Autodesk Inventor part; units mm, degrees
ref_plane "YZ Plane" through (0, 0, 0) normal (1, 0, 0) x (0, 1, 0)
ref_plane "XZ Plane" through (0, 0, 0) normal (0, 1, 0) x (-1, 0, 0)
ref_plane "XY Plane" through (0, 0, 0) normal (0, 0, 1) x (1, 0, 0)
sketch "Sketch1" plane through (0, 0, 0) normal (0, 1, 0) x (-1, 0, 0)
  line L0 (19.2289, 19.6338) -> (19.2289, -32.3662)
  line L1 (17.2289, -34.3662) -> (-13.7711, -34.3662)
  line L2 (-15.7711, -32.3662) -> (-15.7711, -10.826)
  line L3 (-19.7711, -6.826) -> (-35.887, -6.826)
  line L4 (-37.887, -4.826) -> (-37.887, 10.574)
  line L5 (17.2289, 21.6338) -> (-13.3861, 21.6338)
  line L6 (-14.943, 20.8893) -> (-16.2097, 19.3185)
  line L7 (-17.7665, 18.574) -> (-35.887, 18.574)
  line L8 (-16.8101, 12.574) -> (-36.4101, 12.574)
  line L9 (-36.4101, 12.574) -> (-36.4101, 10.174)
  line L10 (-36.4101, 10.174) -> (-16.8101, 10.174)
  line L11 (-16.8101, 10.174) -> (-16.8101, 12.574)
  arc A0 (19.2289, 19.6338) -> (17.2289, 21.6338) centre (17.2289, 19.6338) ccw
  arc A1 (17.2289, -34.3662) -> (19.2289, -32.3662) centre (17.2289, -32.3662) ccw
  arc A2 (-15.7711, -32.3662) -> (-13.7711, -34.3662) centre (-13.7711, -32.3662) ccw
  arc A3 (-15.7711, -10.826) -> (-19.7711, -6.826) centre (-19.7711, -10.826) ccw
  arc A4 (-37.887, -4.826) -> (-35.887, -6.826) centre (-35.887, -4.826) ccw
  arc A5 (-17.7665, 18.574) -> (-16.2097, 19.3185) centre (-17.7665, 20.574) ccw
  arc A6 (-13.3861, 21.6338) -> (-14.943, 20.8893) centre (-13.3861, 19.6338) ccw
  line L12 (-33.327, 18.574) -> (-41.327, 18.574)
  line L13 (-43.327, 16.574) -> (-43.327, 14.574)
  line L14 (-41.327, 12.574) -> (-39.887, 12.574)
  circle A7 centre (-40.327, 15.574) radius 1.5
  arc A8 (-37.887, 10.574) -> (-39.887, 12.574) centre (-39.887, 10.574) ccw
  arc A9 (-43.327, 14.574) -> (-41.327, 12.574) centre (-41.327, 14.574) ccw
  arc A10 (-41.327, 18.574) -> (-43.327, 16.574) centre (-41.327, 16.574) ccw
  circle A11 centre (16.0065, 17.5338) radius 1.5
  circle A12 centre (16.0065, -30.2662) radius 1.5
  circle A13 centre (0.5532, 4.6338) radius 1.5
  line L15 (3.2844, -26.2176) -> (-1.7156, -26.2176)
  line L16 (-1.7156, -26.2176) -> (-1.7156, -23.2176)
  line L17 (-1.7156, -23.2176) -> (3.2844, -23.2176)
  line L18 (3.2844, -23.2176) -> (3.2844, -26.2176)
  line L19 (3.2844, -20.0075) -> (-1.7156, -20.0075)
  line L20 (-1.7156, -20.0075) -> (-1.7156, -17.0075)
  line L21 (-1.7156, -17.0075) -> (3.2844, -17.0075)
  line L22 (3.2844, -17.0075) -> (3.2844, -20.0075)
  point P0 (0, 0)
  point P1 (-43.327, 12.574)
  dimension "d5" = 19.6
  dimension "d6" = 2.4
  dimension "d7" = 17
  dimension "d8" = 6
  dimension "d9" = 56
  dimension "d11" = 2
  dimension "d12" = 4
  dimension "d14" = 3
  dimension "d15" = 2
  dimension "d16" = 3
  dimension "d17" = 35
  dimension "d18" = 3
  dimension "d19" = 3
  dimension "d23" = 5
  dimension "d24" = 3
  dimension "d25" = 5
  dimension "d26" = 3
sketch "Sketch2" plane through (0, 0, 0) normal (0, 1, 0) x (-1, 0, 0)
  point P0 (0, 0)
extrude "Extrusion2" add sketch "Sketch1" along normal blind 3
properties part number "coxa"
Design review of the part built by this model. Coordinates are the model's own, in mm. A direction names the side the tool comes from. Give positions to 0.01 mm unless a question says otherwise; leave off trailing zeros. Write each loop counter-clockwise with the first axis right and the second up, starting at its lowest first coordinate (ties: lowest second). Pieces come first, ordered by that corner, then holes. Notation, with made-up numbers: M 23,70.25 L 48,70.25 A19 cw 48,91.25 Z; hole C 84,41 d7. An arc over 180 degrees is marked long. Answer as a JSON object with one key per item and string values. Group by question number.
1) Clearance check with flat-ended pins moving along their axes: pin 1 Ø2.5 at (x, z) = (-16.01, 17.53) entering from -Y; pin 2 Ø1.5 at (x, y) = (20.5, 2.5) entering from +Z. State where each tip first meets the part, or that it passes through.
2) For line 1 along Z through (x, y) = (-3, 2.05); line 2 along Z through (x, y) = (32, 0.45); line 3 along X through (y, z) = (1.9, -18), list the stretches that pass through material, from the lowest coordinate up.
3) We need section A-A (x = 26.5). Give the boundary of the cut face in (y, z), and give its area (3 significant figures).
4) Tool access review of faces 1 (the face through (26, 1, 12.574)), 2 (the face through (16.892, 1.479, 18.775)), 3 (the face through (41, 1, 12.574)): name each direction out of +Z, -Z, +X, -X, +Y, -Y from which nothing blocks a thin tool from reaching the whole face with its end or side.
5) We need section C-C (y = 0.8). Count the separate pieces of the cut face and the enclosed holes in it, and give its area (3 significant figures).
6) We need section B-B (z = -13). Give the boundary of the cut face in (x, y), and give its area (3 significant figures).
7) We need section D-D (z = -2). Give the boundary of the cut face in (x, y).
8) Mouldability with a two-part tool opening along Z and no side actions: class faces 4 (the face through (-3.284, 1, -25)), 5 (the face through (-16.699, 1.479, -28.935)), 6 (the face through (42.726, 1.479, 13.144)), 7 (the face through (29, 1, 18.574)) as released by +Z, released by -Z, zero draft, split by the parting line, or undercut.
Answer key:
{
 "1": {"pin 1": "passes through", "pin 2": "stops at z = 18.57"},
 "2": {"line 1": "z = -34.37 to -26.22, -23.22 to -20.01, -17.01 to 21.63", "line 2": "z = -6.83 to 10.17, 12.57 to 18.57", "line 3": "x = -19.23 to -3.28, 1.72 to 15.77"},
 "3": {"outline": "M 0,-6.83 L 3,-6.83 L 3,10.17 L 0,10.17 Z; M 0,12.57 L 3,12.57 L 3,18.57 L 0,18.57 Z", "area": "69.0 mm²"},
 "4": {"face 1": "+Y, -Y", "face 2": "+Z, +X, +Y, -Y", "face 3": "-Z, +X, +Y, -Y"},
 "5": {"separate pieces": "1", "enclosed holes": "7", "area": "2,450 mm²"},
 "6": {"outline": "M -19.23,0 L 15.77,0 L 15.77,3 L -19.23,3 Z", "area": "105 mm²"},
 "7": {"outline": "M -19.23,0 L 37.89,0 L 37.89,3 L -19.23,3 Z"},
 "8": {"face 4": "undercut", "face 5": "undercut", "face 6": "released by -Z", "face 7": "released by +Z"}
}
